Build history of the part. All positions in model axes, mm. Face numbers are marked on the shaded views. A direction names the side the tool comes from. Round coordinates to 2 decimals unless told otherwise and drop trailing zeros. Write each loop counter-clockwise with the first axis right and the second up, starting at its lowest first coordinate (ties: lowest second). Pieces come first, ordered by that corner, then holes.
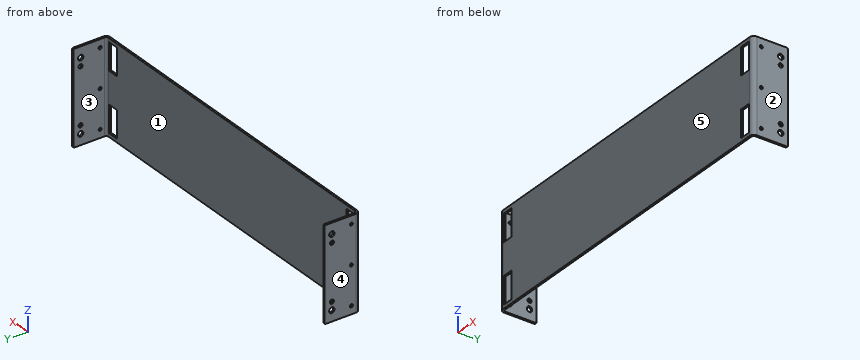
from build123d import *

# Parameters (mm, degrees)
F1_DEPTH = 82.467501
F2_R     = 1.98374
F3_R     = 3.69316
F4_R     = 2.4125
F4_R_2   = 1.8288
F4_R_3   = 1.35255
F5_DEPTH = 308.21884
F6_W     = 9.532925
F6_H     = 24
F7_DEPTH = 31.336894
F8_R     = 0.762


with BuildPart() as f1:
    # F0 (on Top) → F1 (new body)
    with BuildSketch(Plane.XY):
        Polygon((0, 29.627474), (0, 0), (-304.8, 0), (-304.8, 29.627474), (-306.50942, 29.627474), (-306.50942, -1.70942), (1.70942, -1.70942), (1.70942, 29.627474), align=None)
    extrude(amount=F1_DEPTH)

    # F2
    f2_edges = [f1.edges().sort_by_distance(p)[0] for p in [
        (0, 0, 41.23375),
        (-304.8, 0, 41.23375),
    ]]
    fillet(f2_edges, radius=F2_R)

    # F3
    f3_edges = [f1.edges().sort_by_distance(p)[0] for p in [
        (1.70942, -1.70942, 41.23375),
        (-306.50942, -1.70942, 41.23375),
    ]]
    fillet(f3_edges, radius=F3_R)

    # F4 (on face) → F5 (cut, through all)
    with BuildSketch(Plane(origin=(-306.50942, 0, 0), x_dir=(0, -1, 0), z_dir=(-1, 0, 0))):
        with Locations((-23.246224, 9.483746)):
            Circle(F4_R)
        with Locations((-23.246224, 72.983755)):
            Circle(F4_R)
        with Locations((-23.246224, 65.808755)):
            Circle(F4_R_2)
        with Locations((-23.246224, 16.658746)):
            Circle(F4_R_2)
        with Locations((-5.95249, 7.14375)):
            Circle(F4_R_3)
        with Locations((-5.95249, 75.323751)):
            Circle(F4_R_3)
        with Locations((-5.95249, 41.23375)):
            Circle(F4_R_3)
    extrude(amount=-F5_DEPTH, mode=Mode.SUBTRACT)

    # F6 (on face) → F7 (cut, through all)
    with BuildSketch(Plane.XZ.offset(1.70942)):
        with Locations((-7.543952, 15.175)):
            Rectangle(F6_W, F6_H)
        with Locations((-7.543952, 67.292501)):
            Rectangle(F6_W, F6_H)
        with Locations((-297.256048, 67.292501)):
            Rectangle(F6_W, F6_H)
        with Locations((-297.256048, 15.175)):
            Rectangle(F6_W, F6_H)
    extrude(amount=-F7_DEPTH, mode=Mode.SUBTRACT)

    # F8
    f8_edges = [f1.edges().sort_by_distance(p)[0] for p in [
        (0.85471, 29.627474, 82.467501),
        (0.85471, 29.627474, 0),
        (-305.65471, 29.627474, 0),
        (-305.65471, 29.627474, 82.467501),
    ]]
    fillet(f8_edges, radius=F8_R)


solid = f1.part
1) Slice it at D-D (x = -200). Write the cut outline in (y, z).
Results:
outline: (-1.71, 0) - (0, 0) - (0, 82.47) - (-1.71, 82.47) - close
2) Slice it at C-C (z = 49). Write the cut outline in (x, y).
Results:
outline: (-306.51, 1.98) arc R3.69 ccw to (-302.82, -1.71) - (-1.98, -1.71) arc R3.69 ccw to (1.71, 1.98) - (1.71, 29.63) - (0, 29.63) - (0, 1.98) arc R1.98 cw to (-1.98, 0) - (-302.82, 0) arc R1.98 cw to (-304.8, 1.98) - (-304.8, 29.63) - (-306.51, 29.63) - close
3) Slice it at A-A (z = 23). Write the cut outline in (x, y), plus the area to 3 significant figures.
Results:
outline: (-306.51, 1.98) arc R3.69 ccw to (-302.82, -1.71) - (-302.02, -1.71) - (-302.02, 0) - (-302.82, 0) arc R1.98 cw to (-304.8, 1.98) - (-304.8, 29.63) - (-306.51, 29.63) - close; (-292.49, -1.71) - (-12.31, -1.71) - (-12.31, 0) - (-292.49, 0) - close; (-2.78, -1.71) - (-1.98, -1.71) arc R3.69 ccw to (1.71, 1.98) - (1.71, 29.63) - (0, 29.63) - (0, 1.98) arc R1.98 cw to (-1.98, 0) - (-2.78, 0) - close
area: 591 mm2
4) Pin check, flat tips, straight feed: pin 1 Ø0.5 at (y, z) = (-1, 9.5) entering from -X; pin 2 Ø4.5 at (y, z) = (23.25, 72.98) entering from -X; pin 3 Ø0.5 at (x, y) = (-9.5, -0.5) entering from -Z; pin 4 Ø1.4 at (y, z) = (-1, 63.5) entering from -X. Stop position of each tip, or through.
Results:
pin 1: stops at x = -305.3
pin 2: passes through
pin 3: stops at z = 0
pin 4: stops at x = -305.72
5) Slice it at B-B (y = 16.5). Write the cut outline in (x, z), plus the area to 3 significant figures.
Results:
outline: (-306.51, 0) - (-304.8, 0) - (-304.8, 82.47) - (-306.51, 82.47) - close; (0, 0) - (1.71, 0) - (1.71, 82.47) - (0, 82.47) - close
area: 282 mm2
6) Mould opens along X. For the marked faces 3, 4 and 5 say: released by +X, released by -X, zero draft, split by the parting line, or undercut.
Results:
face 3: undercut
face 4: released by -X
face 5: zero draft
7) Which spindle directions (+Z, -Z, +X, -X, +Y, -Y) get a long thin tool onto all of the face, cutting with end or side? Do the marked faces 1 and 2. Say none if no direction does.
Results:
face 1: +Z, -Z, +Y
face 2: +Z, -Z, +X, +Y, -Y
8) Wall check: L1, parallel to X at y = 17, z = 30.5; L2, parallel to Y at x = -192, z = 75.5. Give the ranges that are in metal, low to high.
Results:
L1: x = -306.51 to -304.8, 0 to 1.71
L2: y = -1.71 to 0
